```python
from build123d import *

# Parameters (mm, degrees)
F0_W      = 25.4
F0_H      = 25.4
F1_DEPTH  = 25.4
F5_W      = 87.4159298837
F5_H      = 133.6338296533
F6_DEPTH  = 25.4
F9_W      = 100.1058854163
F9_H      = 223.7386330962
F10_DEPTH = 25.4


with BuildPart() as f1:
    # F0 (on Top) → F1 (new body)
    with BuildSketch(Plane.XY):
        Rectangle(F0_W, F0_H)
    extrude(amount=F1_DEPTH)

    # F5 (on 3pt) → F6 (cut)
    with BuildSketch(Plane(origin=(-7.0819495099, -14.1638990198, 12.0212404911), x_dir=(-0.9344077554, 0.2715776833, -0.2304944873), z_dir=(0.3562052031, 0.7124104062, -0.6046397824))):
        with Locations((19.7420697659, 46.980433166)):
            Rectangle(F5_W, F5_H)
    extrude(amount=-F6_DEPTH, mode=Mode.SUBTRACT)

    # F9 (on 3pt) → F10 (cut)
    with BuildSketch(Plane(origin=(3.6094875517, 3.9343350679, -2.4191651376), x_dir=(-0.7879237292, 0.5245449158, -0.3225350031), z_dir=(0.6157728453, 0.6711913157, -0.4127057314))):
        with Locations((-17.2750819474, 77.5100886822)):
            Rectangle(F9_W, F9_H)
    extrude(amount=F10_DEPTH, mode=Mode.SUBTRACT)


solid = f1.part
```
Work out the finished part from the listing and answer in its coordinate system (mm). Give positions to 0.01 mm unless a question says otherwise; leave off trailing zeros. Order: outer loops, then holes, each group sorted by start corner. A loop starts at its lowest first (then second) coordinate and runs counter-clockwise, first axis right, second up.
1. Section B-B, the plane y = 3.5 is taken. Determine the outline of the cut face in (x, z), and give its area (3 significant figures).
Result sheet:
outline: (-12.7, 0) - (5.7, 0) - (12.7, 10.44) - (12.7, 25.4) - (-12.7, 25.4) - close
area: 609 mm2
2. Straight lines are drawn through the part: L1, parallel to X at y = -9.25, z = 22; L2, parallel to Y at x = 7.5, z = 23.25; L3, parallel to Y at x = 0.25, z = 22.5. For each, find the intervals that lie inside material, in ascending order.
Result sheet:
L1: x = 0.03 to 12.7
L2: y = -11.92 to 12.7
L3: y = -8.94 to 12.7
3. The mould has two halves that part along Z. Classify faces 1 (the flat face through (-5.47, -8.36, 19.81)), 2 (the flat face through (12.7, -3, 15)), 3 (the flat face through (6.2, 7.59, 7.39)): released by +Z, released by -Z, zero draft, split by the parting line, or undercut.
Result sheet:
face 1: released by +Z
face 2: zero draft
face 3: released by -Z
4. Section C-C, the plane x = -1.75 is taken. Determine the outline of the cut face in (y, z) (3 decimals).
Result sheet:
outline: (-12.7, 0) - (10.339, 0) - (12.7, 3.84) - (12.7, 25.4) - (-5.475, 25.4) - (-12.7, 16.887) - close
5. This flat-tipped pin is pushed along its axis until it touches: P1, Ø1, axis at x = -0.5, z = 18.5, coming from the -Y side. Where does it stop, or does it pass through?
Result sheet:
P1: stops at y = -12.45
6. Section D-D, the plane y = -3.5 is taken. Determine the outline of the cut face in (x, z), and give its area (3 significant figures).
Result sheet:
outline: (-12.7, 0) - (12.7, 0) - (12.7, 25.4) - (-5.7, 25.4) - (-12.7, 21.28) - close
area: 631 mm2
7. Section A-A, the plane z = 18.25 is taken. Determine the outline of the cut face in (x, y).
Result sheet:
outline: (-12.7, -6.07) - (0.56, -12.7) - (12.7, -12.7) - (12.7, 8.3) - (7.91, 12.7) - (-12.7, 12.7) - close
